Build history of the part. All positions in model axes, mm. A direction names the side the tool comes from. Give positions to 0.01 mm unless a question says otherwise; leave off trailing zeros. Loops run counter-clockwise (first coordinate to the right, second up) from the corner with the lowest first, then second, coordinate; pieces in that order, holes last. Notation, with made-up numbers: M 30.5,30 L 50.5,30 A23 cw 50.5,57 Z; hole C 72.5,18 d4. An arc over 180 degrees is marked long. Answer in a Markdown table with one row per item. Add a question column.
```python
from build123d import *

# Parameters (mm, degrees)
CUT_EXTRUDE2_START  = -16
SKETCH7_R           = 10.15
SKETCH7_R_2         = 7.15
CUT_EXTRUDE2_DEPTH  = 1
SKETCH10_W          = 5
SKETCH10_H          = 3
CUT_EXTRUDE3_DEPTH  = 40
SKETCH11_R          = 10.15
SKETCH11_R_2        = 7.15
CUT_EXTRUDE4_DEPTH  = 1
CUT_EXTRUDE5_START  = -3
SKETCH13_R          = 10.15
SKETCH13_R_2        = 7.15
CUT_EXTRUDE5_DEPTH  = 1
CUT_EXTRUDE6_START  = -61
SKETCH14_W          = 5
SKETCH14_H          = 3
CUT_EXTRUDE6_DEPTH  = 30
SKETCH15_R          = 6
BOSS_EXTRUDE4_DEPTH = 20
SKETCH16_W          = 3
SKETCH16_H          = 1.5
CUT_EXTRUDE7_DEPTH  = 15
SKETCH17_R          = 6
BOSS_EXTRUDE5_DEPTH = 3
SKETCH18_R          = 6.5
SKETCH18_R_2        = 5.75
CUT_EXTRUDE8_DEPTH  = 1
CUT_EXTRUDE9_START  = -1
SKETCH19_R          = 6.5
SKETCH19_R_2        = 5.75
CUT_EXTRUDE9_DEPTH  = 1


with BuildPart() as part:
    # Sketch5 → Revolve1 (revolve)
    with BuildSketch(Plane(origin=(0, 0, 0), x_dir=(0, 0, -1), z_dir=(1, 0, 0)), mode=Mode.PRIVATE) as revolve1_sk:
        Polygon((0, 0), (0, 6), (12, 6), (12, 7.5), (91, 7.5), (91, 9), (96, 9), (96, 6), (108, 6), (108, 0), align=None)
    revolve(revolve1_sk.sketch.rotate(Axis((0, 0, 0), (0, 0, -1)), 90), axis=Axis((0, 0, 0), (0, 0, -1)))

    # Sketch7 → Cut-Extrude2 (cut)
    with BuildSketch(Plane.XY.offset(CUT_EXTRUDE2_START)):
        Circle(SKETCH7_R)
        Circle(SKETCH7_R_2, mode=Mode.SUBTRACT)
    extrude(amount=-CUT_EXTRUDE2_DEPTH, mode=Mode.SUBTRACT)

    # Sketch10 → Cut-Extrude3 (cut)
    with BuildSketch(Plane.XY.offset(-17)):
        with Locations((0, 7)):
            Rectangle(SKETCH10_W, SKETCH10_H)
    extrude(amount=-CUT_EXTRUDE3_DEPTH, mode=Mode.SUBTRACT)

    # Sketch11 → Cut-Extrude4 (cut)
    with BuildSketch(Plane.XY.offset(-57)):
        Circle(SKETCH11_R)
        Circle(SKETCH11_R_2, mode=Mode.SUBTRACT)
    extrude(amount=-CUT_EXTRUDE4_DEPTH, mode=Mode.SUBTRACT)

    # Sketch13 → Cut-Extrude5 (cut)
    with BuildSketch(Plane.XY.offset(-57).offset(CUT_EXTRUDE5_START)):
        Circle(SKETCH13_R)
        Circle(SKETCH13_R_2, mode=Mode.SUBTRACT)
    extrude(amount=-CUT_EXTRUDE5_DEPTH, mode=Mode.SUBTRACT)

    # Sketch14 → Cut-Extrude6 (cut)
    with BuildSketch(Plane.XY.offset(CUT_EXTRUDE6_START)):
        with Locations((0, 7)):
            Rectangle(SKETCH14_W, SKETCH14_H)
    extrude(amount=-CUT_EXTRUDE6_DEPTH, mode=Mode.SUBTRACT)

    # Sketch15 → Boss-Extrude4 (add)
    with BuildSketch(Plane.XY):
        Circle(SKETCH15_R)
    extrude(amount=BOSS_EXTRUDE4_DEPTH)

    # Sketch16 → Cut-Extrude7 (cut)
    with BuildSketch(Plane.XY.offset(20)):
        with Locations((0, 5.25)):
            Rectangle(SKETCH16_W, SKETCH16_H)
    extrude(amount=-CUT_EXTRUDE7_DEPTH, mode=Mode.SUBTRACT)

    # Sketch17 → Boss-Extrude5 (add)
    with BuildSketch(Plane.XY.offset(20)):
        Circle(SKETCH17_R)
    extrude(amount=BOSS_EXTRUDE5_DEPTH)

    # Sketch18 → Cut-Extrude8 (cut)
    with BuildSketch(Plane(origin=(0, 0, 20), x_dir=(-1, 0, 0), z_dir=(0, 0, -1))):
        Circle(SKETCH18_R)
        Circle(SKETCH18_R_2, mode=Mode.SUBTRACT)
    extrude(amount=-CUT_EXTRUDE8_DEPTH, mode=Mode.SUBTRACT)

    # Sketch19 → Cut-Extrude9 (cut)
    with BuildSketch(Plane.XY.offset(5).offset(CUT_EXTRUDE9_START)):
        Circle(SKETCH19_R)
        Circle(SKETCH19_R_2, mode=Mode.SUBTRACT)
    extrude(amount=CUT_EXTRUDE9_DEPTH, mode=Mode.SUBTRACT)


solid = part.part
```
(1) Pull direction Z, two halves, no side cores. Call faces 1 (the cylindrical face through (-0.93, 7.09, -16.49)), 2 (the cylindrical face through (-0.75, 5.7, 4.49)), 3 (the flat face through (0, 0, 23)), 4 (the cylindrical face through (5.723, -1.802, -102.084)): +Z half, -Z half, draft (parallel to the pull), parting line (faces both ways), or undercut.
(2) Slice it at A-A, the plane z = -30. Give the cut face in (x, y), then the cut area to 3 significant figures.
(3) Pin check, flat tips, straight feed: pin 1 (5 mm diameter, centred on x = -2.5, z = -82.5, fed in from -Y); pin 2 (1.3 mm diameter, centred on y = 6.5, z = -77, fed in from -X); pin 3 (8 mm diameter, centred on y = -6.5, z = -35.5, fed in from -X). Stop position of each tip, or through.
(4) Tool access for faces 5 (the flat face through (0, 4.5, 13)), 6 (the cylindrical face through (-0.93, 7.09, -57.49)), 7 (the cylindrical face through (-6, 0, 22)): list every direction of +Z, -Z, +X, -X, +Y, -Y with a clear straight run to the whole face (end or side of a thin tool).
(5) Wall check: line 1 (X direction, y = 5.75, z = -71.5); line 2 (Z direction, x = 5, y = -5); line 3 (Y direction, x = -2.25, z = -32.5). Give the ranges that are in metal, low to high.
Solution:
| question | item | result |
|---|---|---|
| 1 | face 1 | undercut |
| 1 | face 2 | undercut |
| 1 | face 3 | +Z half |
| 1 | face 4 | draft |
| 2 | outline | M -2.5,5.5 L -2.5,7.07 A7.5 ccw long 2.5,7.07 L 2.5,5.5 Z |
| 2 | area | 167 mm^2 |
| 3 | pin 1 | y = -7.5 |
| 3 | pin 2 | x = -4.69 |
| 3 | pin 3 | x = -7.07 |
| 4 | face 5 | +Y |
| 4 | face 6 | none |
| 4 | face 7 | +Z |
| 5 | line 1 | -4.82 to -2.5, 2.5 to 4.82 |
| 5 | line 2 | -96 to -12 |
| 5 | line 3 | -7.15 to 5.5 |
